For this review, take the finished solid that the model builds, in its own axes (mm). A direction names the side the tool comes from. Coordinates: 2 decimals unless noted, no trailing zeros. Order: outer loops, then holes, each group sorted by start corner. A loop starts at its lowest first (then second) coordinate and runs counter-clockwise, first axis right, second up. Notation, with made-up numbers: (38.5, 47.25) -> (53.5, 47.25) arc R16 cw to (53.5, 64.25) -> close; hole circle Ø7 at (-3, 61). An arc over 180 degrees is marked (long way). Answer as a JSON object with one key per item and string values. Group by question number.
1) Add section D-D, the plane y = -2.25. Write out the cut boundary in (x, z).
2) Machinability: for faces 1 (the cylindrical face through (0.36, -15.66, 6.76)), 2 (the flat face through (1, 3.281, 4)), which of the approach directions +Z, -Z, +X, -X, +Y, -Y give a long, thin tool a straight path to every point of the face, cutting with its end or side? Answer none if there is none.
3) Draft analysis for pull direction Y (two halves, no side actions). For faces 3 (the cylindrical face through (0.576, -14.683, 3.042)), 4 (the flat face through (1, -16.719, 4)), 5 (the cylindrical face through (0.576, -1.683, 3.042)), 6 (the flat face through (8.401, -7, 4)), state which applies: +Y half, -Y half, draft (parallel to the pull), parting line (faces both ways), or undercut.
4) Add section B-B, the plane x = 1.75. Write out the cut boundary in (y, z), then the cut area to 3 significant figures.
5) Wall thickness on L1, parallel to Y at x = 1.25, z = 5.75; L2, parallel to Z at x = -0.5, y = -14.5; L3, parallel to Y at x = 0, z = 1: over which ranges is each line inside the solid? List them lowest first.
6) Add section C-C, the plane z = 5. Write out the cut boundary in (x, y).
7) Add section A-A, the plane y = -14. Write out the cut boundary in (x, z), then the cut area to 3 significant figures.
8) For pin 1 (1.5 mm diameter, centred on x = 0.5, y = -14, fed in from +Z); pin 2 (3.5 mm diameter, centred on x = 0.9, y = -13.22, fed in from -Z), all flat-tipped, find the tip position at first contact; note any pin that passes through.
from build123d import *

# Parameters (mm, degrees)
IZIM1_W                     = 15
IZIM1_H                     = 20
Y_KSEKLIK_EKSTR_ZYON1_DEPTH = 7.5
IZIM2_R                     = 1.5
KES_EKSTR_ZYON1_DEPTH       = 7.5
IZIM3_R                     = 2.5
KES_EKSTR_ZYON2_DEPTH       = 1.5


with BuildPart() as part:
    # Çizim1 → Yükseklik-Ekstrüzyon1 (new body)
    with BuildSketch(Plane.XY):
        with Locations((0.901187863, -6.71875)):
            Rectangle(IZIM1_W, IZIM1_H)
    extrude(amount=Y_KSEKLIK_EKSTR_ZYON1_DEPTH)

    # Çizim2 → Kes-Ekstrüzyon1 (cut)
    with BuildSketch(Plane.XY.offset(7.5)):
        with Locations((0.901187863, -0.21875)):
            Circle(IZIM2_R)
        with Locations((0.901187863, -13.21875)):
            Circle(IZIM2_R)
    extrude(amount=-KES_EKSTR_ZYON1_DEPTH, mode=Mode.SUBTRACT)

    # Çizim3 → Kes-Ekstrüzyon2 (cut)
    with BuildSketch(Plane.XY.offset(7.5)):
        with Locations((0.901187863, -0.21875)):
            Circle(IZIM3_R)
        with Locations((0.901187863, -13.21875)):
            Circle(IZIM3_R)
    extrude(amount=-KES_EKSTR_ZYON2_DEPTH, mode=Mode.SUBTRACT)


solid = part.part
Output values:
{
 "1": {"outline": "(-6.6, 0) -> (8.4, 0) -> (8.4, 7.5) -> (2.36, 7.5) -> (2.36, 6) -> (-0.56, 6) -> (-0.56, 7.5) -> (-6.6, 7.5) -> close"},
 "2": {"face 1": "+Z", "face 2": "+Z, -Z, +X, -X, +Y"},
 "3": {"face 3": "undercut", "face 4": "-Y half", "face 5": "undercut", "face 6": "draft"},
 "4": {"outline": "(-16.72, 0) -> (-14.46, 0) -> (-14.46, 6) -> (-15.57, 6) -> (-15.57, 7.5) -> (-16.72, 7.5) -> close; (-11.98, 0) -> (-1.46, 0) -> (-1.46, 6) -> (-2.57, 6) -> (-2.57, 7.5) -> (-10.87, 7.5) -> (-10.87, 6) -> (-11.98, 6) -> close; (1.02, 0) -> (3.28, 0) -> (3.28, 7.5) -> (2.13, 7.5) -> (2.13, 6) -> (1.02, 6) -> close", "area": "106 mm²"},
 "5": {"L1": "y = -16.72 to -14.68, -11.76 to -1.68, 1.24 to 3.28", "L2": "z = 0 to 6", "L3": "y = -16.72 to -14.42, -12.02 to -1.42, 0.98 to 3.28"},
 "6": {"outline": "(-6.6, -16.72) -> (8.4, -16.72) -> (8.4, 3.28) -> (-6.6, 3.28) -> close; hole circle Ø3 at (0.9, -13.22); hole circle Ø3 at (0.9, -0.22)"},
 "7": {"outline": "(-6.6, 0) -> (-0.38, 0) -> (-0.38, 6) -> (-1.47, 6) -> (-1.47, 7.5) -> (-6.6, 7.5) -> close; (2.18, 0) -> (8.4, 0) -> (8.4, 7.5) -> (3.28, 7.5) -> (3.28, 6) -> (2.18, 6) -> close", "area": "90.0 mm²"},
 "8": {"pin 1": "stops at z = 6", "pin 2": "stops at z = 0"}
}
